Design review of the part shown in the three views and the two pictorial views. Dimensions are in mm from the part's minimum x, y and z. A direction names the side the tool comes from. Give positions to 0.01 mm unless a question says otherwise; leave off trailing zeros. Loops run counter-clockwise (first coordinate to the right, second up) from the corner with the lowest first, then second, coordinate; pieces in that order, holes last.
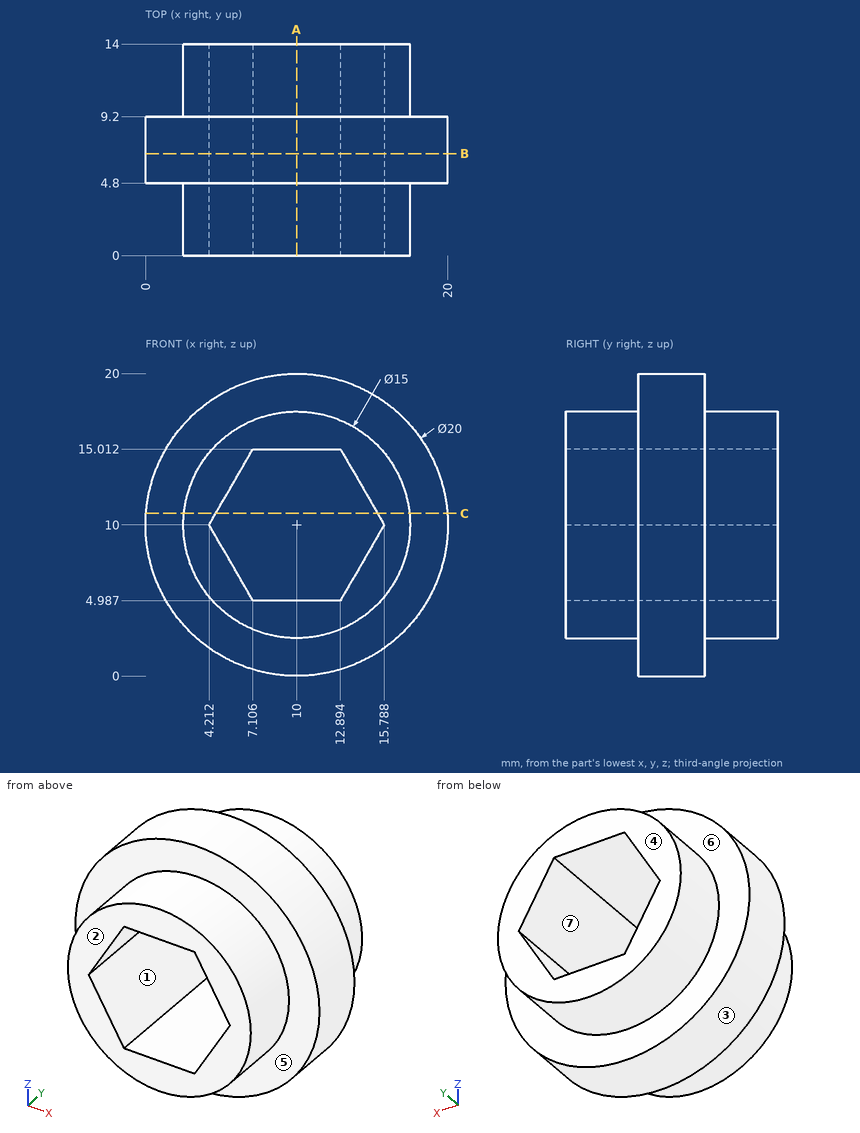
Q1. Insertion check: pin 1 (4 mm diameter, centred on y = 4.5, z = 4, fed in from +X) (1 decimal); pin 2 (1 mm diameter, centred on y = 6, z = 6.5, fed in from -X); pin 3 (5 mm diameter, centred on y = 12, z = 15, fed in from -X); pin 4 (4.5 mm diameter, centred on x = 11.5, y = 8.5, fed in from +Z). Each pin has a flat end and moves straight along its axis. Give the tip position at first contact, or say it passes through.
Results:
pin 1: stops at x = 19.2
pin 2: stops at x = 0.46
pin 3: stops at x = 2.93
pin 4: stops at z = 20
Q2. Tool access review of the marked faces 4, 5, 6 and 7: name each direction out of +Z, -Z, +X, -X, +Y, -Y from which nothing blocks a thin tool from reaching the whole face with its end or side.
Results:
face 4: +Z, -Z, +X, -X, +Y
face 5: -Y
face 6: +Y
face 7: +Y, -Y
Q3. Take a section at A-A (x = 10). Give the boundary of the cut face in (y, z).
Results:
outline: (0, 2.5) - (4.8, 2.5) - (4.8, 0) - (9.2, 0) - (9.2, 2.5) - (14, 2.5) - (14, 4.99) - (0, 4.99) - close; (0, 15.01) - (14, 15.01) - (14, 17.5) - (9.2, 17.5) - (9.2, 20) - (4.8, 20) - (4.8, 17.5) - (0, 17.5) - close
Q4. Take a section at C-C (z = 10.75). Give the boundary of the cut face in (x, y) (1 decimal).
Results:
outline: (0, 4.8) - (2.5, 4.8) - (2.5, 0) - (4.6, 0) - (4.6, 14) - (2.5, 14) - (2.5, 9.2) - (0, 9.2) - close; (15.4, 0) - (17.5, 0) - (17.5, 4.8) - (20, 4.8) - (20, 9.2) - (17.5, 9.2) - (17.5, 14) - (15.4, 14) - close
Q5. Wall thickness on line 1 (Z direction, x = 10, y = 12.25); line 2 (Z direction, x = 10, y = 6.5); line 3 (Y direction, x = 19.25, z = 12): over which ranges is each line inside the solid? List them lowest first.
Results:
line 1: z = 2.5 to 4.99, 15.01 to 17.5
line 2: z = 0 to 4.99, 15.01 to 20
line 3: y = 4.8 to 9.2
Q6. Draft analysis for pull direction Z (two halves, no side actions). For the marked faces 1, 2 and 3, state which applies: pulls with the +Z half, pulls with the -Z half, needs draft (parallel to the pull), parting line crosses it, or undercut.
Results:
face 1: undercut
face 2: needs draft
face 3: parting line crosses it
Q7. Take a section at B-B (y = 6.75). Give the boundary of the cut face in (x, z), plus the area to 3 significant figures.
Results:
outline: circle Ø20 at (10, 10); hole (4.21, 10) - (7.11, 4.99) - (12.89, 4.99) - (15.79, 10) - (12.89, 15.01) - (7.11, 15.01) - close
area: 227 mm2
